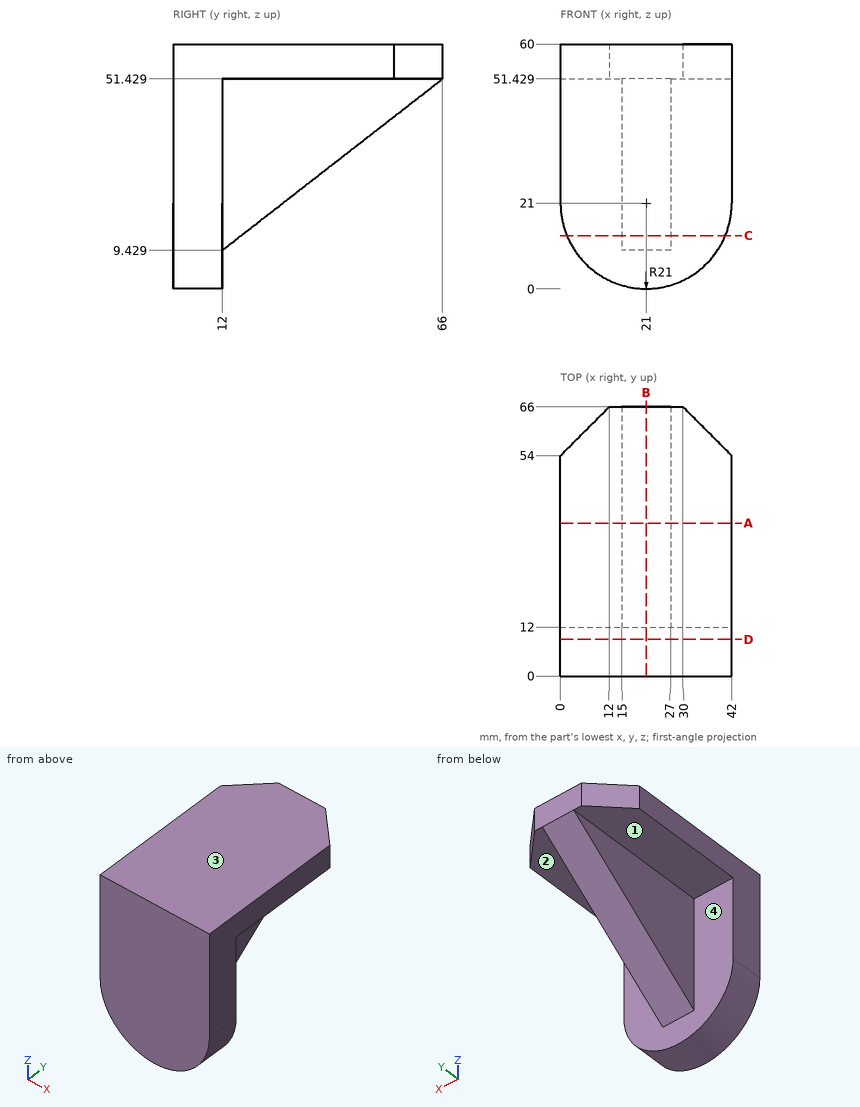
Check sheet for the drawn part. Datum: minimum x, y, z corner. Units: mm. A direction names the side the tool comes from. Coordinates: 2 decimals unless noted, no trailing zeros. Write each loop counter-clockwise with the first axis right and the second up, starting at its lowest first coordinate (ties: lowest second). Pieces come first, ordered by that corner, then holes. Notation, with made-up numbers: M 65.25,-20 L 112.25,-20 A32 cw 112.25,19 Z; hole C 20.5,-39.5 d2. An arc over 180 degrees is marked long. Use a Markdown table: item, result.
Q1. Sectioned sample at B-B, the plane x = 21. Record the boundary of the cut face in (y, z), plus the area to 3 significant figures.
Reply:
| item | result |
|---|---|
| outline | M 0,0 L 12,0 L 12,9.43 L 66,51.43 L 66,60 L 0,60 Z |
| area | 2,320 mm² |
Q2. Sectioned sample at C-C, the plane z = 13. Record the boundary of the cut face in (x, y).
Reply:
| item | result |
|---|---|
| outline | M 1.58,0 L 40.42,0 L 40.42,12 L 27,12 L 27,16.59 L 15,16.59 L 15,12 L 1.58,12 Z |
Q3. Sectioned sample at A-A, the plane y = 37.5. Record the boundary of the cut face in (x, z).
Reply:
| item | result |
|---|---|
| outline | M 0,51.43 L 15,51.43 L 15,29.26 L 27,29.26 L 27,51.43 L 42,51.43 L 42,60 L 0,60 Z |
Q4. Thickness scan on line 1 (Z direction, x = 36, y = 44); line 2 (Y direction, x = 11.5, z = 48.5); line 3 (X direction, y = 50, z = 42.5). Record the ranges inside material, lowest first.
Reply:
| item | result |
|---|---|
| line 1 | z = 51.43 to 60 |
| line 2 | y = 0 to 12 |
| line 3 | x = 15 to 27 |
Q5. Sectioned sample at D-D, the plane y = 9. Record the boundary of the cut face in (x, z), plus the area to 3 significant figures.
Reply:
| item | result |
|---|---|
| outline | M 0,21 A21 ccw 42,21 L 42,60 L 0,60 Z |
| area | 2,330 mm² |
Q6. Set-up check for the marked faces 1, 2, 3 and 4: record each of +Z, -Z, +X, -X, +Y, -Y from which the full face is reachable in a straight line by a thin tool's end or side.
Reply:
| item | result |
|---|---|
| face 1 | -Z, -X, +Y |
| face 2 | -Z, +X, +Y |
| face 3 | +Z, +X, -X, +Y, -Y |
| face 4 | -Z, +Y |
Q7. Go/stop test with flat-tipped pins: P1, Ø10, axis at x = 30.5, y = 33.5, coming from the -Z side (1 decimal); P2, Ø12.5, axis at y = 42.5, z = 37, coming from the +X side; P3, Ø12, axis at x = 23.5, y = 16.5, coming from the -Z side. Record where each tip stops, or that it passes through.
Reply:
| item | result |
|---|---|
| P1 | stops at z = 23.4 |
| P2 | stops at x = 27 |
| P3 | stops at z = 0 |
